Read the model definition and answer for the solid it produces. Units are mm, in the model's axes. Face numbers are marked on the shaded views. Give positions to 0.01 mm unless a question says otherwise; leave off trailing zeros. One line per item, written item: value. Start each with the question number.
from build123d import *
from build123d.topology import SkipClean

# Parameters (mm, degrees)
SKETCH1_R           = 123.825
BOSS_EXTRUDE1_DEPTH = 10
SKETCH4_R           = 111.825
CUT_EXTRUDE1_DEPTH  = 5.5
CUT_EXTRUDE1_DRAFT  = -30
SKETCH5_R           = 111.825
CUT_EXTRUDE2_DEPTH  = 5.5
CUT_EXTRUDE2_DRAFT  = -30
SKETCH6_R           = 20
BOSS_EXTRUDE2_DEPTH = 4
BOSS_EXTRUDE2_TAPER = 30
SKETCH9_R           = 20
BOSS_EXTRUDE3_DEPTH = 4
BOSS_EXTRUDE3_TAPER = 30
CUT_EXTRUDE4_DEPTH  = 24
SKETCH11_R          = 123.825
SKETCH11_R_2        = 116.325
BOSS_EXTRUDE4_DEPTH = 0.25
BOSS_EXTRUDE5_START = 0.25
SKETCH13_R          = 123.825
SKETCH13_R_2        = 116.325
BOSS_EXTRUDE5_DEPTH = 0.25


with BuildPart() as part:
    # Sketch1 → Boss-Extrude1 (new, symmetric)
    with BuildSketch(Plane.XY):
        Circle(SKETCH1_R)
    extrude(amount=BOSS_EXTRUDE1_DEPTH, both=True)


with BuildPart() as cut_extrude1_tool:
    # Sketch4 → Cut-Extrude1 (with draft: the straight prism first)
    with BuildSketch(Plane.XY.offset(10)):
        Circle(SKETCH4_R)
    extrude(amount=-CUT_EXTRUDE1_DEPTH)
    # Cut-Extrude1: the draft: its side faces are tilted about the plane it starts from
    cut_extrude1_sides = [cut_extrude1_tool.faces().sort_by_distance(p)[0] for p in [
        (-111.825, 0, 7.25),
    ]]
    draft(cut_extrude1_sides, Plane.XY.offset(10), CUT_EXTRUDE1_DRAFT)


with BuildPart() as part_1:
    add(part.part)

    # Cut-Extrude1: cut by cut_extrude1_tool
    add(cut_extrude1_tool.part, mode=Mode.SUBTRACT)


with BuildPart() as cut_extrude2_tool:
    # Sketch5 → Cut-Extrude2 (with draft: the straight prism first)
    with BuildSketch(Plane(origin=(0, 0, -10), x_dir=(-1, 0, 0), z_dir=(0, 0, -1))):
        Circle(SKETCH5_R)
    extrude(amount=-CUT_EXTRUDE2_DEPTH)
    # Cut-Extrude2: the draft: its side faces are tilted about the plane it starts from
    cut_extrude2_sides = [cut_extrude2_tool.faces().sort_by_distance(p)[0] for p in [
        (111.825, 0, -7.25),
    ]]
    draft(cut_extrude2_sides, Plane(origin=(0, 0, -10), x_dir=(-1, 0, 0), z_dir=(0, 0, -1)), CUT_EXTRUDE2_DRAFT)


with BuildPart() as part_2:
    add(part_1.part)

    # Cut-Extrude2: cut by cut_extrude2_tool
    add(cut_extrude2_tool.part, mode=Mode.SUBTRACT)

    # Sketch6 → Boss-Extrude2 (add)
    with BuildSketch(Plane.XY.offset(4.5)):
        Circle(SKETCH6_R)
    extrude(amount=BOSS_EXTRUDE2_DEPTH, taper=BOSS_EXTRUDE2_TAPER)

    # Sketch9 → Boss-Extrude3 (add)
    with BuildSketch(Plane(origin=(0, 0, -4.5), x_dir=(-1, 0, 0), z_dir=(0, 0, -1))):
        Circle(SKETCH9_R)
    extrude(amount=BOSS_EXTRUDE3_DEPTH, taper=BOSS_EXTRUDE3_TAPER)

    # Sketch10 → Cut-Extrude4 (cut)
    with BuildSketch(Plane(origin=(0, 0, -8.5), x_dir=(-1, 0, 0), z_dir=(0, 0, -1))):
        Polygon((7.450577941, -3.554421662), (6.803508425, 4.675178938), (-0.647069515, 8.2296006), (-7.450577941, 3.554421662), (-6.803508425, -4.675178938), (0.647069515, -8.2296006), align=None)
    extrude(amount=-CUT_EXTRUDE4_DEPTH, mode=Mode.SUBTRACT)

    # Sketch11 → Boss-Extrude4 (add)
    with BuildSketch(Plane(origin=(0, 0, -10), x_dir=(-1, 0, 0), z_dir=(0, 0, -1))):
        Circle(SKETCH11_R)
        Circle(SKETCH11_R_2, mode=Mode.SUBTRACT)
    extrude(amount=BOSS_EXTRUDE4_DEPTH)

    # Sketch13 → Boss-Extrude5 (add)
    with SkipClean():  # the faces are left unmerged after this step: merging them gives an invalid solid
        with BuildSketch(Plane.XY.offset(10).offset(BOSS_EXTRUDE5_START)):
            with Locations(Location((0, 0, 0), (0, 0, 180))):
                Circle(SKETCH13_R)
            with Locations(Location((0, 0, 0), (0, 0, 180))):
                Circle(SKETCH13_R_2, mode=Mode.SUBTRACT)
        extrude(amount=-BOSS_EXTRUDE5_DEPTH)


solid = part_2.part
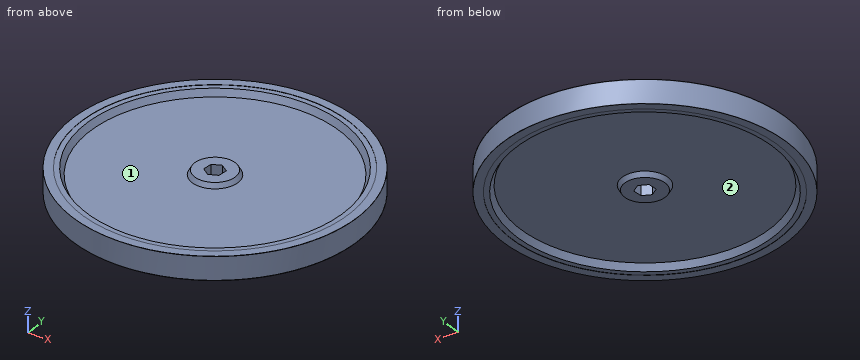
Item 1: Consider L1, parallel to Y at x = 0, z = -10.1 (3 decimals); L2, parallel to Z at x = -17.5, y = 35; L3, parallel to X at y = -72.5, z = 7. Determine where each line is inside the solid, lowest interval first. Write a range as [from, to].
Item 2: Determine the mould class of the marked faces 1 and 2 for opening direction Y: pulls with the +Y half, pulls with the -Y half, needs draft (parallel to the pull), parting line crosses it, or undercut.
Item 3: Flat-ended cylindrical pins translate along their axes: pin 1 (10 mm diameter, centred on x = -38, z = -6, fed in from -Y); pin 2 (6 mm diameter, centred on y = 8, z = 2.5, fed in from -X); pin 3 (10.5 mm diameter, centred on x = 8.5, y = -4.5, fed in from +Z). Find the tip coordinate at first contact, or state that the pin passes through.
Computed values:
1. L1: [-123.825, -116.325], [116.325, 123.825]
1. L2: [-4.5, 4.5]
1. L3: [-100.38, -82.85], [82.85, 100.38]
2. face 1: undercut
2. face 2: undercut
3. pin 1: y = -119.35
3. pin 2: x = -123.72
3. pin 3: z = 8.5
